Check sheet for the modelled part. Datum: model origin and axes. Units: mm. Face numbers are marked on the shaded views. A direction names the side the tool comes from. Round coordinates to 2 decimals unless told otherwise and drop trailing zeros. Loops run counter-clockwise (first coordinate to the right, second up) from the corner with the lowest first, then second, coordinate; pieces in that order, holes last. Notation, with made-up numbers: (-34.75, 73) - (-7.75, 73) arc R16 cw to (-7.75, 102) - close; hole circle Ø8 at (39.5, -28.75). An arc over 180 degrees is marked (long way). Put each result on its own line as item: value. Start each with the question number.
Item 1: Material ranges on line 1 along Z through (x, y) = (130, -15); line 2 along Z through (x, y) = (-130, -25); line 3 along X through (y, z) = (-32, 375.5), recorded low to high.
Item 2: Tool access check on the marked faces 4, 5 and 6. Record the directions out of +Z, -Z, +X, -X, +Y, -Y that give a thin tool (end or side, any length) a straight path to the whole face; none if there is none.
Item 3: Section check C-C, the plane y = 80. Record the cut outline in (x, z).
Item 4: Draft check along Z on the marked faces 1, 2 and 3. Enter one of: pulls with the +Z half, pulls with the -Z half, needs draft (parallel to the pull), parting line crosses it, or undercut.
Item 5: Gauge pin test, flat ends, axial feed: pin 1 Ø1 at (x, z) = (60, 153.5) entering from +Y; pin 2 Ø12 at (x, y) = (-124.5, -11.5) entering from +Z; pin 3 Ø3 at (y, z) = (-16.5, 172.5) entering from -X. Record the tip position at first contact, or that the pin passes through.
Item 6: Section check A-A, the plane x = -51.5. Record the cut outline in (y, z).
Item 7: Section check D-D, the plane x = 29. Record the cut outline in (y, z).
Item 8: Section check B-B, the plane z = 34.5. Record the cut outline in (x, y), and give its area (3 significant figures).
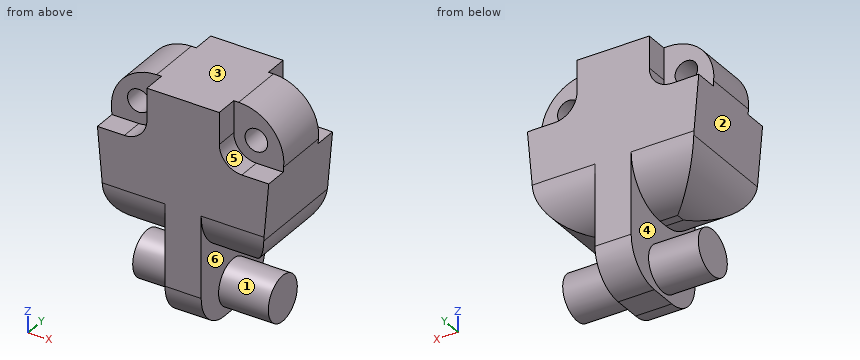
from build123d import *

# Parameters (mm, degrees)
F1_DEPTH      = 110
F2_W          = 300
F2_H          = 50
F4_W          = 120
F4_H          = 50
F5_DEPTH      = 120
F6_R          = 50
F7_R          = 100
F8_R          = 25
F9_DEPTH      = 110.001
F9_DEPTH_BACK = 110.001
F10_R         = 80


with BuildPart() as f1:
    # F0 (on Front) → F1 (new body, symmetric)
    with BuildSketch(Plane.XZ):
        Polygon((-40, -60), (0, -60), (40, -60), (40, 100), (170.2538544012, 100), (200, 440), (0, 440), (-200, 440), (-170.2538544012, 100), (-40, 100), align=None)
    extrude(amount=F1_DEPTH, both=True)

    # F2 (on Front) → F3 (revolve)
    with BuildSketch(Plane.XZ):
        with Locations((0, 25)):
            Rectangle(F2_W, F2_H)
    revolve(axis=Axis((165.973843012, 0, 0), (1, 0, 0)))

    # F4 (on face) → F5 (cut)
    with BuildSketch(Plane.XY.offset(440)):
        with Locations((140, -85)):
            Rectangle(F4_W, F4_H)
        with Locations((140, 85)):
            Rectangle(F4_W, F4_H)
        with Locations((-140, 85)):
            Rectangle(F4_W, F4_H)
        with Locations((-140, -85)):
            Rectangle(F4_W, F4_H)
    extrude(amount=-F5_DEPTH, mode=Mode.SUBTRACT)

    # F6
    f6_edges = [f1.edges().sort_by_distance(p)[0] for p in [
        (80, -85, 320),
        (-80, -85, 320),
        (-80, 85, 320),
        (80, 85, 320),
    ]]
    fillet(f6_edges, radius=F6_R)

    # F7
    f7_edges = [f1.edges().sort_by_distance(p)[0] for p in [
        (200, 0, 440),
        (-200, 0, 440),
        (105.126927, -110, 100),
        (170.253854, 0, 100),
        (105.126927, 110, 100),
        (-105.126927, 110, 100),
        (-105.126927, -110, 100),
        (-170.253854, 0, 100),
    ]]
    fillet(f7_edges, radius=F7_R)

    # F8 (on Front) → F9 (cut, two sides)
    with BuildSketch(Plane.XZ) as f9_sk:
        with Locations((130, 370)):
            Circle(F8_R)
        with Locations((-130, 370)):
            Circle(F8_R)
    extrude(amount=-F9_DEPTH, mode=Mode.SUBTRACT)
    extrude(f9_sk.sketch, amount=F9_DEPTH_BACK, mode=Mode.SUBTRACT)

    # F10
    f10_edges = [f1.edges().sort_by_distance(p)[0] for p in [
        (0, -110, -60),
        (0, 110, -60),
    ]]
    fillet(f10_edges, radius=F10_R)


solid = f1.part
Check result:
1. line 1: -47.7 to 47.7, 114.21 to 345, 395 to 432.03
1. line 2: -43.3 to 43.3, 114.21 to 345, 395 to 432.03
1. line 3: -184.36 to -154.39, -105.61 to 105.61, 154.39 to 184.36
2. face 4: -X
2. face 5: +Z, +X, -Y
2. face 6: +X
3. outline: (-189.5, 320) - (-178.24, 191.28) arc R100 ccw to (-148.62, 128.59) - (-40, 128.59) - (-40, -42.45) - (40, -42.45) - (40, 128.59) - (148.62, 128.59) arc R100 ccw to (178.24, 191.28) - (189.5, 320) - (130, 320) arc R50 cw to (80, 370) - (80, 440) - (-80, 440) - (-80, 370) arc R50 cw to (-130, 320) - close
4. face 1: undercut
4. face 2: pulls with the -Z half
4. face 3: pulls with the +Z half
5. pin 1: y = 98.79
5. pin 2: z = 436.11
5. pin 3: x = -175.18
6. outline: (-110, 200) arc R100 ccw to (-10, 100) - (10, 100) arc R100 ccw to (110, 200) - (110, 440) - (-110, 440) - close; circle Ø100 at (0, 0)
7. outline: (-110, 20) arc R80 ccw to (-30, -60) - (30, -60) arc R80 ccw to (110, 20) - (110, 440) - (-110, 440) - close
8. outline: (-150, -36.19) - (-40, -36.19) - (-40, -110) - (40, -110) - (40, -36.19) - (150, -36.19) - (150, 36.19) - (40, 36.19) - (40, 110) - (-40, 110) - (-40, 36.19) - (-150, 36.19) - close
8. area: 33,500 mm²
